Job drawing, mm, ordinate dimensions from the low corner. One solid piece. A direction names the side the tool comes from. Give positions to 0.01 mm unless a question says otherwise; leave off trailing zeros. Loops run counter-clockwise (first coordinate to the right, second up) from the corner with the lowest first, then second, coordinate; pieces in that order, holes last. Notation, with made-up numbers: (58, -25) -> (81, -25) arc R22 ccw to (81, -6) -> close; hole circle Ø1 at (-3.5, -24). An arc over 180 degrees is marked (long way). Answer as a JSON object with one key per item and string values. Group by question number.
Q1. Wall check: probe 1 along X at (y, z) = (15.5, 1.75); probe 2 along Y at (x, z) = (24.05, 15); probe 3 along Y at (x, z) = (17.75, 21.5). Give the ranges that are in metal, low to high. Write a range as from..to.
Q2. Band-saw the part on B-B, the plane y = 25. Write the cut outline in (x, z).
Q3. Band-saw the part on A-A, the plane z = 15. Write the cut outline in (x, y).
Q4. Drop flat-ended pins along their axis: pin 1 (5 mm diameter, centred on x = 14.5, y = 17, fed in from -Z); pin 2 (9 mm diameter, centred on y = 24.5, z = 9, fed in from -X); pin 3 (6 mm diameter, centred on y = 24.5, z = 21.5, fed in from +X); pin 4 (2.5 mm diameter, centred on x = 14, z = 9.5, fed in from +Y). Give the stop position or say it passes through.
Q5. Two-plate mould, pull along Y, no slides. Class the marked faces 4, 5 and 6: pulls with the +Y half, pulls with the -Y half, needs draft (parallel to the pull), parting line crosses it, or undercut.
Q6. Band-saw the part on D-D, the plane z = 23.75. Write the cut outline in (x, y), plus the area to 3 significant figures.
Q7. Tool access for the marked faces 1, 2 and 3: list every direction of +Z, -Z, +X, -X, +Y, -Y with a clear straight run to the whole face (end or side of a thin tool).
Q8. Band-saw the part on C-C, the plane x = 10. Write the cut outline in (y, z).
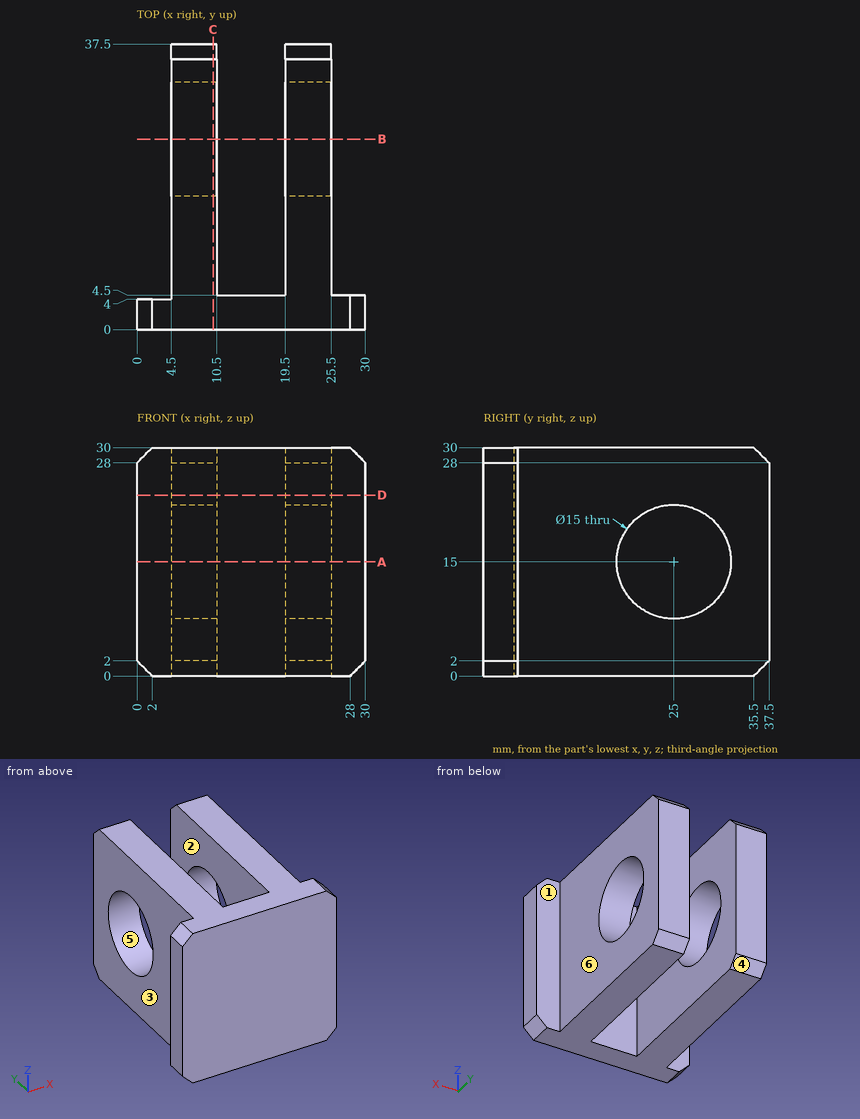
Worked answers:
{
 "1": {"probe 1": "4.5..10.5, 19.5..25.5", "probe 2": "0..17.5, 32.5..37.5", "probe 3": "0..4.5"},
 "2": {"outline": "(4.5, 0) -> (10.5, 0) -> (10.5, 7.5) -> (4.5, 7.5) -> close; (4.5, 22.5) -> (10.5, 22.5) -> (10.5, 30) -> (4.5, 30) -> close; (19.5, 0) -> (25.5, 0) -> (25.5, 7.5) -> (19.5, 7.5) -> close; (19.5, 22.5) -> (25.5, 22.5) -> (25.5, 30) -> (19.5, 30) -> close"},
 "3": {"outline": "(0, 0) -> (30, 0) -> (30, 4.5) -> (25.5, 4.5) -> (25.5, 17.5) -> (19.5, 17.5) -> (19.5, 4.5) -> (10.5, 4.5) -> (10.5, 17.5) -> (4.5, 17.5) -> (4.5, 4) -> (0, 4) -> close; (4.5, 32.5) -> (10.5, 32.5) -> (10.5, 37.5) -> (4.5, 37.5) -> close; (19.5, 32.5) -> (25.5, 32.5) -> (25.5, 37.5) -> (19.5, 37.5) -> close"},
 "4": {"pin 1": "through", "pin 2": "x = 4.5", "pin 3": "x = 25.5", "pin 4": "y = 4.5"},
 "5": {"face 4": "pulls with the +Y half", "face 5": "undercut", "face 6": "needs draft"},
 "6": {"outline": "(0, 0) -> (30, 0) -> (30, 4.5) -> (25.5, 4.5) -> (25.5, 37.5) -> (19.5, 37.5) -> (19.5, 4.5) -> (10.5, 4.5) -> (10.5, 37.5) -> (4.5, 37.5) -> (4.5, 4) -> (0, 4) -> close", "area": "529 mm2"},
 "7": {"face 1": "+Z, -Z, +X, +Y", "face 2": "+Z, -Z, +Y", "face 3": "+Z, -Z, -X, +Y"},
 "8": {"outline": "(0, 0) -> (35.5, 0) -> (37.5, 2) -> (37.5, 28) -> (35.5, 30) -> (0, 30) -> close; hole circle Ø15 at (25, 15)"}
}
